Could you check a few things on this model? Use its own coordinates, in mm. Coordinates: 2 decimals unless noted, no trailing zeros. Loops run counter-clockwise (first coordinate to the right, second up) from the corner with the lowest first, then second, coordinate; pieces in that order, holes last. Notation, with made-up numbers: (53, 89) - (109, 89) arc R27 ccw to (109, 105) - close; hole circle Ø4 at (-39.75, 9.5). An arc over 180 degrees is marked (long way). One line per question, with ' | ' between items. Start each with the question number.
1. We'd pull the mould along Z, two halves only. Please class faces 1 (the cylindrical face through (0.45, 1.06, 1.43)), 2 (the flat face through (3.3, 1, 0)), 3 (the flat face through (0, 1, 3.3)): pulls with the +Z half, pulls with the -Z half, needs draft (parallel to the pull), parting line crosses it, or undercut.
2. I want a section at A-A, the plane z = 0. Write out the boundary of the cut face in (x, y).
3. I want a section at C-C, the plane y = 0.85. Write out the boundary of the cut face in (x, z).
4. I want a section at B-B, the plane x = 0. Write out the boundary of the cut face in (y, z), then the cut area to 3 significant figures.
5. Please list where these lines run through material, in increasing order: L1, parallel to X at y = 0.8, z = 0; L2, parallel to X at y = 0.1, z = 1; L3, parallel to Z at x = 0.5, y = 0.35. Write a range as [from, to].
from build123d import *

# Parameters (mm, degrees)
SKETCH_1_W          = 6.6
SKETCH_1_H          = 6.6
EXTRUDE_1_DEPTH     = 2
SKETCH_2_R          = 1.5
CUT_EXTRUDE_1_DEPTH = 2
FILLET_1_R          = 0.2
FILLET_2_R          = 0.1


with BuildPart() as part:
    # 草图1 → 凸台-拉伸1 (new body)
    with BuildSketch(Plane(origin=(0, 0, 0), x_dir=(1, 0, 0), z_dir=(0, 1, 0))):
        Rectangle(SKETCH_1_W, SKETCH_1_H)
    extrude(amount=EXTRUDE_1_DEPTH)

    # 草图2 → 切除-拉伸1 (cut)
    with BuildSketch(Plane(origin=(0, 2, 0), x_dir=(1, 0, 0), z_dir=(0, 1, 0))):
        with Locations(Location((0, 0, 0), (0, 0, 270))):
            Circle(SKETCH_2_R)
    extrude(amount=-CUT_EXTRUDE_1_DEPTH, mode=Mode.SUBTRACT)

    # 圆角1
    fillet_1_edges = [part.edges().sort_by_distance(p)[0] for p in [
        (-3.3, 1, -3.3),
        (3.3, 1, -3.3),
        (3.3, 1, 3.3),
        (-3.3, 1, 3.3),
    ]]
    fillet(fillet_1_edges, radius=FILLET_1_R)

    # 圆角2
    fillet_2_edges = [part.edges().sort_by_distance(p)[0] for p in [
        (0, 0, -1.5),
        (-3.3, 0, 0),
        (-3.3, 2, 0),
        (0, 0, -3.3),
        (3.3, 0, 0),
        (0, 0, 3.3),
        (-3.241421356, 0, 3.241421356),
        (3.241421356, 0, 3.241421356),
        (3.241421356, 0, -3.241421356),
        (-3.241421356, 0, -3.241421356),
        (0, 2, -3.3),
        (0, 2, 3.3),
        (3.3, 2, 0),
        (-3.241421356, 2, 3.241421356),
        (3.241421356, 2, 3.241421356),
        (3.241421356, 2, -3.241421356),
        (-3.241421356, 2, -3.241421356),
    ]]
    fillet(fillet_2_edges, radius=FILLET_2_R)


solid = part.part
Results are:
1) face 1: undercut | face 2: needs draft | face 3: pulls with the +Z half
2) outline: (-3.3, 0.1) arc R0.1 ccw to (-3.2, 0) - (-1.6, 0) arc R0.1 ccw to (-1.5, 0.1) - (-1.5, 2) - (-3.2, 2) arc R0.1 ccw to (-3.3, 1.9) - close; (1.5, 0.1) arc R0.1 ccw to (1.6, 0) - (3.2, 0) arc R0.1 ccw to (3.3, 0.1) - (3.3, 1.9) arc R0.1 ccw to (3.2, 2) - (1.5, 2) - close
3) outline: (-3.3, -3.1) arc R0.2 ccw to (-3.1, -3.3) - (3.1, -3.3) arc R0.2 ccw to (3.3, -3.1) - (3.3, 3.1) arc R0.2 ccw to (3.1, 3.3) - (-3.1, 3.3) arc R0.2 ccw to (-3.3, 3.1) - close; hole circle Ø3 at (0, 0)
4) outline: (0, -3.2) arc R0.1 ccw to (0.1, -3.3) - (1.9, -3.3) arc R0.1 ccw to (2, -3.2) - (2, -1.5) - (0.1, -1.5) arc R0.1 ccw to (0, -1.6) - close; (0, 1.6) arc R0.1 ccw to (0.1, 1.5) - (2, 1.5) - (2, 3.2) arc R0.1 ccw to (1.9, 3.3) - (0.1, 3.3) arc R0.1 ccw to (0, 3.2) - close | area: 7.19 mm2
5) L1: x = [-3.3, -1.5], [1.5, 3.3] | L2: x = [-3.3, -1.12], [1.12, 3.3] | L3: z = [-3.3, -1.41], [1.41, 3.3]
